The model under review builds one solid part; all positions refer to its coordinate system, in mm. A direction names the side the tool comes from. Coordinates: 2 decimals unless noted, no trailing zeros. Loops run counter-clockwise (first coordinate to the right, second up) from the corner with the lowest first, then second, coordinate; pieces in that order, holes last. Notation, with made-up numbers: (31.25, -33.5) - (80.25, -33.5) arc R20 ccw to (80.25, 0.5) - close; hole circle Ø2 at (-24, 20.5). An arc over 180 degrees is marked (long way). Answer in a Markdown table with one row per item. Add a question column.
(1) Mouldability with a two-part tool opening along Z and no side actions: class faces 5 (the flat face through (-3, 0, 3)), 6 (the cylindrical face through (-3.01, -13.95, 59.68)), 7 (the flat face through (-3, -8, 63.5)) as +Z half, -Z half, draft (parallel to the pull), parting line (faces both ways), or undercut.
(2) We need section C-C on z = 34. Write out the cut boundary in (x, y), plus the area to 3 significant figures.
(3) For P1, Ø2, axis at x = -3.175, z = 58.42, coming from the -Y side; P2, Ø3, axis at x = -2, z = 43, coming from the +Y side, all flat-tipped, find the tip position at first contact; note any pin that passes through.
(4) For line 1 along Z through (x, y) = (-0.75, -0.25); line 2 along Z through (x, y) = (-0.5, -6.5); line 3 along Y through (x, z) = (-6, 40), list the stretches that pass through material, from the lowest coordinate up.
(5) We need section A-A on y = -6. Write out the cut boundary in (x, z), plus the area to 3 significant figures.
(6) We need section B-B on x = -2.5. Write out the cut boundary in (y, z).
(7) Machinability: for faces 1 (the flat face through (-3, -8, 2.54)), 2 (the flat face through (-3, -1, 5.08)), 3 (the flat face through (-3, -8, 0)), 4 (the cylindrical face through (-2.9, -13.95, 3.84)), which of the approach directions +Z, -Z, +X, -X, +Y, -Y give a long, thin tool a straight path to every point of the face, cutting with its end or side? Answer none if there is none.
from build123d import *

# Parameters (mm, degrees)
F0_W     = 6.35
F0_H     = 15.24
F1_DEPTH = 63.5
F2_W     = 10.16
F2_H     = 58.42
F3_DEPTH = 25.4
F4_W     = 5.08
F4_H     = 53.34
F5_DEPTH = 25.4
F6_R     = 1.27
F7_DEPTH = 25.4


with BuildPart() as f1:
    # F0 (on Top) → F1 (new body)
    with BuildSketch(Plane.XY):
        with Locations((-3.175, -7.62)):
            Rectangle(F0_W, F0_H)
    extrude(amount=F1_DEPTH)

    # F2 (on face) → F3 (cut)
    with BuildSketch(Plane(origin=(-6.35, 0, 0), x_dir=(0, -1, 0), z_dir=(-1, 0, 0))):
        with Locations((7.62, 31.75)):
            Rectangle(F2_W, F2_H)
    extrude(amount=-F3_DEPTH, mode=Mode.SUBTRACT)

    # F4 (on face) → F5 (cut)
    with BuildSketch(Plane(origin=(-6.35, 0, 0), x_dir=(0, -1, 0), z_dir=(-1, 0, 0))):
        with Locations((1.636012, 31.75)):
            Rectangle(F4_W, F4_H)
    extrude(amount=-F5_DEPTH, mode=Mode.SUBTRACT)

    # F6 (on face) → F7 (cut)
    with BuildSketch(Plane(origin=(0, -12.7, 0), x_dir=(-1, 0, 0), z_dir=(0, 1, 0))):
        with Locations((3.175, 5.08)):
            Circle(F6_R)
        with Locations((3.175, 58.42)):
            Circle(F6_R)
    extrude(amount=-F7_DEPTH, mode=Mode.SUBTRACT)


solid = f1.part
Outcome:
| question | item | result |
|---|---|---|
| 1 | face 5 | draft |
| 1 | face 6 | undercut |
| 1 | face 7 | +Z half |
| 2 | outline | (-6.35, -15.24) - (0, -15.24) - (0, -12.7) - (-6.35, -12.7) - close |
| 2 | area | 16.1 mm² |
| 3 | P1 | y = -2.54 |
| 3 | P2 | y = -12.7 |
| 4 | line 1 | 0 to 5.08, 58.42 to 63.5 |
| 4 | line 2 | 0 to 2.54, 60.96 to 63.5 |
| 4 | line 3 | -15.24 to -12.7 |
| 5 | outline | (-6.35, 0) - (0, 0) - (0, 2.54) - (-6.35, 2.54) - close; (-6.35, 60.96) - (0, 60.96) - (0, 63.5) - (-6.35, 63.5) - close |
| 5 | area | 32.3 mm² |
| 6 | outline | (-15.24, 0) - (0, 0) - (0, 5.08) - (-2.54, 5.08) - (-2.54, 2.54) - (-12.7, 2.54) - (-12.7, 4) - (-15.24, 4) - close; (-15.24, 6.16) - (-12.7, 6.16) - (-12.7, 57.34) - (-15.24, 57.34) - close; (-15.24, 59.5) - (-12.7, 59.5) - (-12.7, 60.96) - (-2.54, 60.96) - (-2.54, 58.42) - (0, 58.42) - (0, 63.5) - (-15.24, 63.5) - close |
| 7 | face 1 | +X, -X |
| 7 | face 2 | +X, -X, +Y |
| 7 | face 3 | -Z, +X, -X, +Y, -Y |
| 7 | face 4 | -Y |
